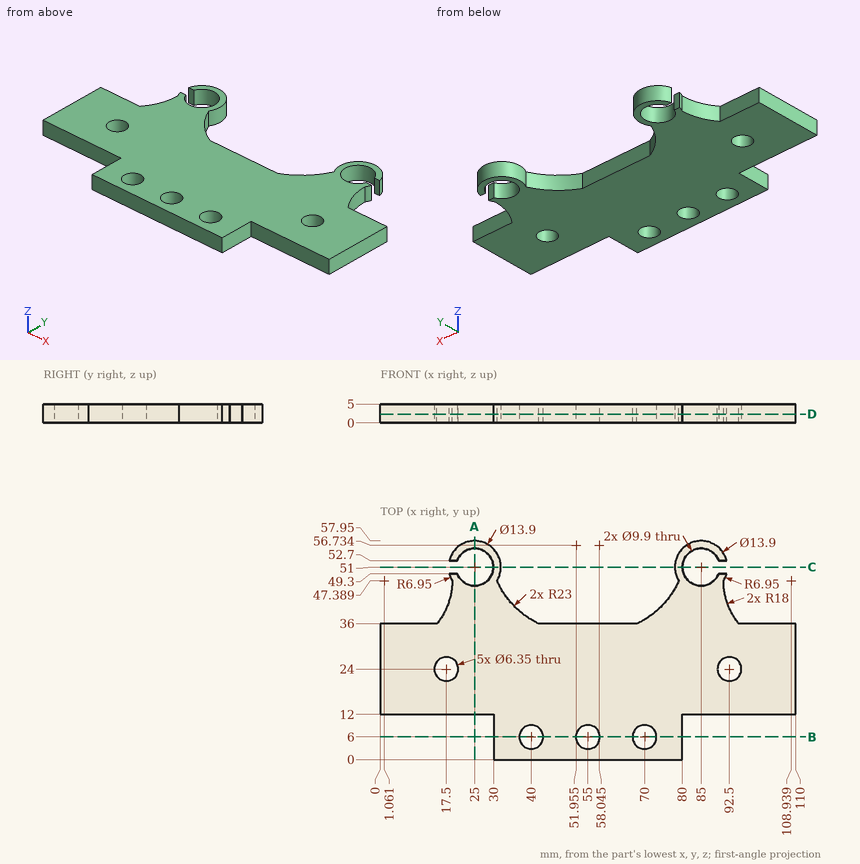
Geometry: see drawing. Coordinates: mm, zero at the bounding-box minimum. Give positions to 0.01 mm unless a question says otherwise; leave off trailing zeros. Write each loop counter-clockwise with the first axis right and the second up, starting at its lowest first coordinate (ties: lowest second). Pieces come first, ordered by that corner, then holes. Notation, with made-up numbers: M -25.5,67 L -14.5,67 A21 cw -14.5,79 Z; hole C 84,-29.5 d4. An arc over 180 degrees is marked long. Return JSON: item names as keys, results as strings. Group by question number.
1) Cut plane D-D, the plane z = 2.35. Give the number of separate pieces and of enclosed holes in the cut face, then the cut area to 3 significant figures.
2) Cut plane A-A, the plane x = 25. Output: boundary loops of the cut face in (y, z).
3) Ray query, L1, parallel to Y at x = 25, z = 2.1; L2, parallel to X at y = 7, z = 1.2 (1 decimal); L3, parallel to X at y = 53, z = 4.35 (1 decimal). Return the intervals inside material, ascending.
4) Cut plane B-B, the plane y = 6. Output: boundary loops of the cut face in (x, z) (1 decimal).
5) First-contact query: pin 1 Ø1 at (x, z) = (90.5, 3.5) entering from -Y; pin 2 Ø2.5 at (y, z) = (7.5, 2) entering from +X; pin 3 Ø4 at (x, y) = (17.5, 24) entering from +Z; pin 4 Ø1.5 at (x, z) = (54, 1.5) entering from +Y. Flat tips, straight axial feed; report the tip coordinate or a pass-through.
6) Cut plane C-C, the plane y = 51. Output: boundary loops of the cut face in (x, z), then the cut area to 3 significant figures.
Data:
{
 "1": {"separate pieces": "1", "enclosed holes": "5", "area": "3,560 mm²"},
 "2": {"outline": "M 12,0 L 46.05,0 L 46.05,5 L 12,5 Z; M 55.95,0 L 57.95,0 L 57.95,5 L 55.95,5 Z"},
 "3": {"L1": "y = 12 to 46.05, 55.95 to 57.95", "L2": "x = 30 to 37, 43 to 52, 58 to 67, 73 to 80", "L3": "x = 18.3 to 20.5, 29.5 to 31.7, 78.3 to 80.5, 89.5 to 91.7"},
 "4": {"outline": "M 30,0 L 36.8,0 L 36.8,5 L 30,5 Z; M 43.2,0 L 51.8,0 L 51.8,5 L 43.2,5 Z; M 58.2,0 L 66.8,0 L 66.8,5 L 58.2,5 Z; M 73.2,0 L 80,0 L 80,5 L 73.2,5 Z"},
 "5": {"pin 1": "stops at y = 12", "pin 2": "stops at x = 80", "pin 3": "passes through", "pin 4": "stops at y = 36"},
 "6": {"outline": "M 29.95,0 L 31.95,0 L 31.95,5 L 29.95,5 Z; M 78.05,0 L 80.05,0 L 80.05,5 L 78.05,5 Z", "area": "20.0 mm²"}
}
